For this review, take the finished solid that the model builds, in its own axes (mm). Face numbers are marked on the shaded views. A direction names the side the tool comes from. Coordinates: 2 decimals unless noted, no trailing zeros. Write each loop counter-clockwise with the first axis right and the second up, starting at its lowest first coordinate (ties: lowest second). Pieces come first, ordered by that corner, then holes. Notation, with made-up numbers: (-2.75, 46.5) - (49.25, 46.5) arc R20 cw to (49.25, 82.5) - close; hole circle Ø2 at (53.5, 19.25). An arc over 180 degrees is marked (long way). Write each question's results on one line, items separated by ' | '.
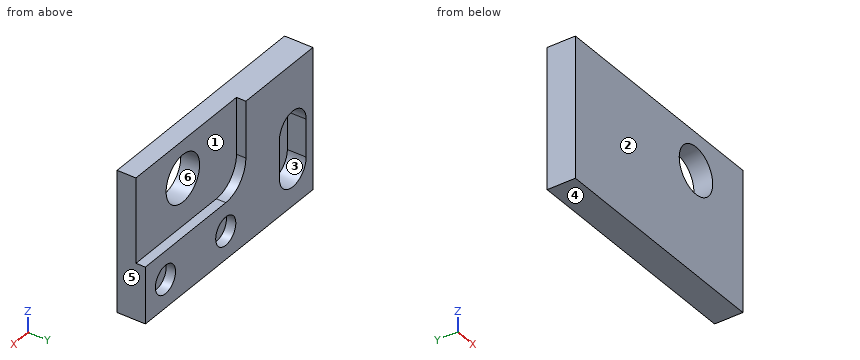
from build123d import *

# Parameters (mm, degrees)
SKETCH2_W           = 250
SKETCH2_H           = 150
BOSS_EXTRUDE1_DEPTH = 30
CUT_EXTRUDE2_DEPTH  = 20
SKETCH3_5_R         = 15
CUT_EXTRUDE3_DEPTH  = 10
SKETCH3_6_R         = 25
CUT_EXTRUDE4_DEPTH  = 149.828760661
SKETCH3_7_R         = 25
CUT_EXTRUDE5_DEPTH  = 10


with BuildPart() as part:
    # Sketch2 → Boss-Extrude1 (new body)
    with BuildSketch(Plane(origin=(0, 0, 0), x_dir=(1, 0, 0), z_dir=(0, 1, 0))):
        Rectangle(SKETCH2_W, SKETCH2_H)
    extrude(amount=-BOSS_EXTRUDE1_DEPTH)

    # Sketch3 → Cut-Extrude2 (cut)
    with BuildSketch(Plane(origin=(0, 0, 0), x_dir=(1, 0, 0), z_dir=(0, 1, 0))):
        with BuildLine():
            Line((-75, 35), (-75, -5))
            ThreePointArc((-75, -5), (-95, -25), (-115, -5))
            Line((-115, -5), (-115, 35))
            ThreePointArc((-115, 35), (-95, 55), (-75, 35))
        make_face()
    extrude(amount=-CUT_EXTRUDE2_DEPTH, mode=Mode.SUBTRACT)

    # Sketch3_5 → Cut-Extrude3 (cut)
    with BuildSketch(Plane(origin=(0, 0, 0), x_dir=(1, 0, 0), z_dir=(0, 1, 0))):
        with Locations(Location((5, 45, 0), (0, 0, 270))):
            Circle(SKETCH3_5_R)
        with Locations(Location((95, 45, 0), (0, 0, 270))):
            Circle(SKETCH3_5_R)
    extrude(amount=-CUT_EXTRUDE3_DEPTH, mode=Mode.SUBTRACT)

    # Sketch3_6 → Cut-Extrude4 (cut, through all)
    with BuildSketch(Plane(origin=(0, 0, 0), x_dir=(1, 0, 0), z_dir=(0, 1, 0))):
        with Locations(Location((55, -35, 0), (0, 0, 270))):
            Circle(SKETCH3_6_R)
    extrude(amount=-CUT_EXTRUDE4_DEPTH, mode=Mode.SUBTRACT)

    # Sketch3_7 → Cut-Extrude5 (cut)
    with BuildSketch(Plane(origin=(0, 0, 0), x_dir=(1, 0, 0), z_dir=(0, 1, 0))):
        with BuildLine():
            Line((-25, -75), (125, -75))
            Line((125, -75), (125, 15))
            Line((125, 15), (5, 15))
            ThreePointArc((5, 15), (-16.213203436, 6.213203436), (-25, -15))
            Line((-25, -15), (-25, -75))
        make_face()
        with Locations(Location((55, -35, 0), (0, 0, 270))):
            Circle(SKETCH3_7_R, mode=Mode.SUBTRACT)
    extrude(amount=-CUT_EXTRUDE5_DEPTH, mode=Mode.SUBTRACT)


solid = part.part
Q1. Take a section at D-D on x = -95. State the section outline as (y, z) points.
Results found:
outline: (-30, -75) - (0, -75) - (0, -55) - (-20, -55) - (-20, 25) - (0, 25) - (0, 75) - (-30, 75) - close
Q2. Wall thickness on line 1 along X through (y, z) = (-15.25, 35); line 2 along Y through (x, z) = (85, 37.5); line 3 along X through (y, z) = (-6.25, -21.5): over which ranges is each line inside the solid? List them lowest first. Write a range as from..to.
Results found:
line 1: -125..30, 80..125 | line 2: -30..-10 | line 3: -125..-115, -75..125
Q3. For pin 1 (3 mm diameter, centred on y = -2.5, z = 50, fed in from +X); pin 2 (9 mm diameter, centred on x = 95, z = -47.5, fed in from +Y), all flat-tipped, find the tip position at first contact; note any pin that passes through.
Results found:
pin 1: x = -25 | pin 2: y = -10
Q4. Take a section at C-C on z = -18.5. State the section outline as (x, y) points, plus the area to 3 significant figures.
Results found:
outline: (-125, -30) - (125, -30) - (125, 0) - (-75, 0) - (-75, -20) - (-115, -20) - (-115, 0) - (-125, 0) - close | area: 6,700 mm2
Q5. For the marked faces 1, 2 and 3, list the 3-axis set-ups (+Z, -Z, +X, -X, +Y, -Y) from which the entire face can be reached by the end or side of a thin tool; tool diameter is ignored.
Results found:
face 1: +Z, +X, +Y | face 2: +Z, -Z, +X, -X, -Y | face 3: +Y
Q6. Take a section at B-B on y = -22.75. State the section outline as (x, z) points.
Results found:
outline: (-125, -75) - (125, -75) - (125, 75) - (-125, 75) - close; hole circle Ø50 at (55, 35)
Q7. Mouldability with a two-part tool opening along X and no side actions: class the marked faces 4, 5 and 6 as pulls with the +X half, pulls with the -X half, needs draft (parallel to the pull), parting line crosses it, or undercut.
Results found:
face 4: needs draft | face 5: pulls with the +X half | face 6: undercut
Q8. Take a section at A-A on x = 55. State the section outline as (y, z) points, plus the area to 3 significant figures.
Results found:
outline: (-30, -75) - (0, -75) - (0, -15) - (-10, -15) - (-10, 10) - (-30, 10) - close; (-30, 60) - (-10, 60) - (-10, 75) - (-30, 75) - close | area: 2,600 mm2
